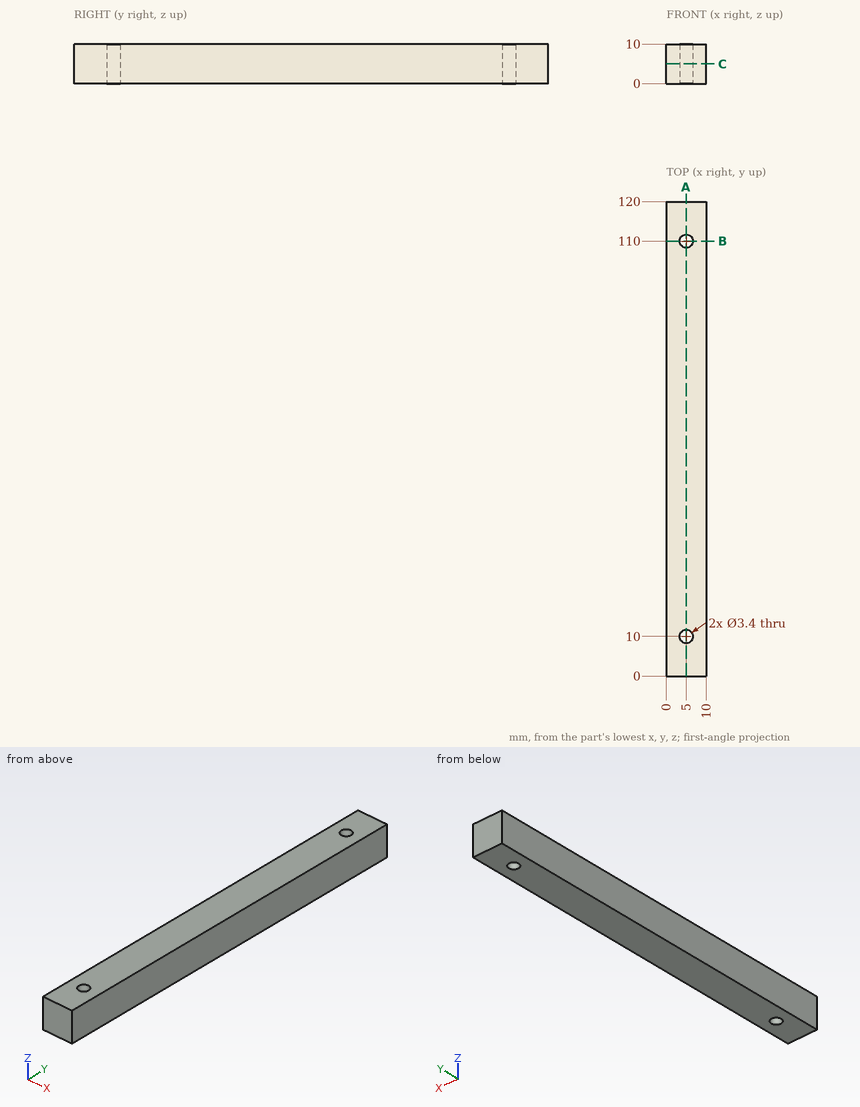
Geometry check sheet. Reference: drawing and pictorial views, mm from the part's lowest x, y, z. Coordinates: 2 decimals unless noted, no trailing zeros. Write each loop counter-clockwise with the first axis right and the second up, starting at its lowest first coordinate (ties: lowest second). Pieces come first, ordered by that corner, then holes.
Item 1: Depth check by flat-ended pin: pin 1 Ø2 at (x, y) = (5, 110) entering from +Z. Enter the tip coordinate at first touch or a pass-through.
Numbers:
pin 1: passes through
Item 2: Cross-section at C-C on z = 5. Record the boundary of the cut face in (x, y), then the cut area to 3 significant figures.
Numbers:
outline: (0, 0) - (10, 0) - (10, 120) - (0, 120) - close; hole circle Ø3.4 at (5, 10); hole circle Ø3.4 at (5, 110)
area: 1,180 mm2
Item 3: Scan lines: probe 1 along Y at (x, z) = (5, 4); probe 2 along X at (y, z) = (110, 6); probe 3 along Y at (x, z) = (6.25, 9). Record each from-to range of solid material in increasing order.
Numbers:
probe 1: y = 0 to 8.3, 11.7 to 108.3, 111.7 to 120
probe 2: x = 0 to 3.3, 6.7 to 10
probe 3: y = 0 to 8.85, 11.15 to 108.85, 111.15 to 120
Item 4: Cross-section at B-B on y = 110. Record the boundary of the cut face in (x, z), then the cut area to 3 significant figures.
Numbers:
outline: (0, 0) - (3.3, 0) - (3.3, 10) - (0, 10) - close; (6.7, 0) - (10, 0) - (10, 10) - (6.7, 10) - close
area: 66.0 mm2
Item 5: Cross-section at A-A on x = 5. Record the boundary of the cut face in (y, z).
Numbers:
outline: (0, 0) - (8.3, 0) - (8.3, 10) - (0, 10) - close; (11.7, 0) - (108.3, 0) - (108.3, 10) - (11.7, 10) - close; (111.7, 0) - (120, 0) - (120, 10) - (111.7, 10) - close
